Source: CAD feature listing. Evaluate the final solid. Frame: model axes, mm. A direction names the side the tool comes from. Round coordinates to 2 decimals unless told otherwise and drop trailing zeros. Loops run counter-clockwise (first coordinate to the right, second up) from the corner with the lowest first, then second, coordinate; pieces in that order, holes last. Notation, with made-up numbers: M 3,22.25 L 62,22.25 A13 cw 62,44.25 Z; hole C 34.5,16.25 d10. An arc over 180 degrees is marked long. Answer as CSV lines item,"result". Start each with the question number.
```python
from build123d import *

# Parameters (mm, degrees)
SKETCH1_W           = 10
SKETCH1_H           = 15.2
BOSS_EXTRUDE1_DEPTH = 1
SKETCH1_8_W         = 10
SKETCH1_8_H         = 15.2
SKETCH1_8_W_2       = 8.44
SKETCH1_8_H_2       = 13.64
BOSS_EXTRUDE2_DEPTH = 1
SKETCH1_9_RX        = 6.016925947
SKETCH1_9_RY        = 3.157568793
BOSS_EXTRUDE3_DEPTH = 0.5
FILLET1_R           = 2


with BuildPart() as part:
    # Sketch1 (on Front Plane) → Boss-Extrude1 (new body)
    with BuildSketch(Plane.XY):
        with Locations((5, 7.6)):
            Rectangle(SKETCH1_W, SKETCH1_H)
    extrude(amount=BOSS_EXTRUDE1_DEPTH)

    # Sketch1<8> (on Front Plane) → Boss-Extrude2 (add)
    with BuildSketch(Plane.XY):
        with Locations((5, 7.6)):
            Rectangle(SKETCH1_8_W, SKETCH1_8_H)
        with Locations((5, 7.6)):
            Rectangle(SKETCH1_8_W_2, SKETCH1_8_H_2, mode=Mode.SUBTRACT)
    extrude(amount=-BOSS_EXTRUDE2_DEPTH)

    # Sketch1<9> (on Front Plane) → Boss-Extrude3 (add)
    # profile 1 of 3: a face of its own
    with BuildSketch(Plane.XY):
        with Locations(Location((5, 7.6), (0, 0, -120.316314342))):
            Ellipse(SKETCH1_9_RX, SKETCH1_9_RY)
        with BuildLine():
            Line((5.55192436, 7.939742657), (5.714255538, 7.749614835))
            ThreePointArc((5.714255538, 7.749614835), (5.903370184, 7.16725844), (5.625306277, 6.621746036))
            Line((5.625306277, 6.621746036), (4.673505596, 5.809098397))
            Line((4.673505596, 5.809098397), (5.102260043, 5.306926538))
            Line((5.102260043, 5.306926538), (3.276812461, 5.306926538))
            Line((3.276812461, 5.306926538), (3.562960201, 7.109807107))
            Line((3.562960201, 7.109807107), (3.991714649, 6.607635249))
            Line((3.991714649, 6.607635249), (5.55192436, 7.939742657))
        make_face(mode=Mode.SUBTRACT)
        with BuildLine():
            Line((4.44807564, 7.260257343), (4.285744462, 7.450385165))
            ThreePointArc((4.285744462, 7.450385165), (4.096629816, 8.03274156), (4.374693723, 8.578253964))
            Line((4.374693723, 8.578253964), (5.326494404, 9.390901603))
            Line((5.326494404, 9.390901603), (4.897739957, 9.893073462))
            Line((4.897739957, 9.893073462), (6.723187539, 9.893073462))
            Line((6.723187539, 9.893073462), (6.437039799, 8.090192893))
            Line((6.437039799, 8.090192893), (6.008285351, 8.592364751))
            Line((6.008285351, 8.592364751), (4.44807564, 7.260257343))
        make_face(mode=Mode.SUBTRACT)
    # profile 2 of 3: a face of its own
    with BuildSketch(Plane.XY):
        with BuildLine():
            add(Edge.make_bspline(
                [(9.22, 11.980450807), (5, 22.611600433), (0.78, 6.751239794)],
                knots=[2.731060957, 2.731060957, 2.731060957, 5.172488647, 5.172488647, 5.172488647], degree=2, weights=[1, 0.342975287, 1]))
            Line((9.22, 11.980450807), (9.22, 14.42))
            Line((9.22, 14.42), (0.78, 14.42))
            Line((0.78, 14.42), (0.78, 6.751239794))
        make_face()
        with BuildLine():
            Line((1.807963278, 12.267050426), (2.573541086, 12.912762773))
            Line((2.573541086, 12.912762773), (2.629548837, 12.846358141))
            ThreePointArc((2.629548837, 12.846358141), (2.72234926, 12.554615255), (2.581675695, 12.282702073))
            Line((2.581675695, 12.282702073), (2.125075804, 11.897591397))
            Line((2.125075804, 11.897591397), (2.341285421, 11.641246159))
            Line((2.341285421, 11.641246159), (1.436292724, 11.641246159))
            Line((1.436292724, 11.641246159), (1.578739925, 12.538825176))
            Line((1.578739925, 12.538825176), (1.807963278, 12.267050426))
        make_face(mode=Mode.SUBTRACT)
        with BuildLine():
            Line((2.79925212, 13.230809928), (2.013248175, 12.570380578))
            Line((2.013248175, 12.570380578), (1.941775235, 12.655443444))
            ThreePointArc((1.941775235, 12.655443444), (1.849520441, 12.947359327), (1.99070215, 13.219009018))
            Line((1.99070215, 13.219009018), (2.47045985, 13.622119038))
            Line((2.47045985, 13.622119038), (2.272289715, 13.857969409))
            Line((2.272289715, 13.857969409), (3.166035288, 13.857969409))
            Line((3.166035288, 13.857969409), (3.036644718, 12.948279301))
            Line((3.036644718, 12.948279301), (2.79925212, 13.230809928))
        make_face(mode=Mode.SUBTRACT)
    # profile 3 of 3: a face of its own
    with BuildSketch(Plane.XY):
        with BuildLine():
            Line((0.78, 0.78), (9.22, 0.78))
            Line((9.22, 0.78), (9.22, 8.448760206))
            add(Edge.make_bspline(
                [(1.745579435, 2.034365319), (6.736770522, -0.884158057), (9.22, 8.448760206)],
                knots=[0, 0, 0, 2.030895994, 2.030895994, 2.030895994], degree=2, weights=[1, 0.527239314, 1]))
            add(Edge.make_bspline(
                [(0.78, 3.219549193), (1.100794809, 2.411393361), (1.745579435, 2.034365319)],
                knots=[5.872653611, 5.872653611, 5.872653611, 6.283185307, 6.283185307, 6.283185307], degree=2, weights=[1, 0.979006832, 1]))
            Line((0.78, 3.219549193), (0.78, 0.78))
        make_face()
        with BuildLine():
            Line((7.056197058, 2.135669885), (7.291696407, 1.863373763))
            Line((7.291696407, 1.863373763), (8.063431346, 2.521185925))
            Line((8.063431346, 2.521185925), (8.112322941, 2.464655019))
            ThreePointArc((8.112322941, 2.464655019), (8.208731591, 2.174084541), (8.071438446, 1.900448977))
            Line((8.071438446, 1.900448977), (7.601212367, 1.493766963))
            Line((7.601212367, 1.493766963), (7.828929297, 1.230469263))
            Line((7.828929297, 1.230469263), (6.912689643, 1.230469263))
            Line((6.912689643, 1.230469263), (7.056197058, 2.135669885))
        make_face(mode=Mode.SUBTRACT)
        with BuildLine():
            Line((8.277665846, 2.828924058), (7.517372897, 2.16210975))
            Line((7.517372897, 2.16210975), (7.461453822, 2.225867947))
            ThreePointArc((7.461453822, 2.225867947), (7.36303426, 2.515763479), (7.498428218, 2.790343716))
            Line((7.498428218, 2.790343716), (7.969285134, 3.203308389))
            Line((7.969285134, 3.203308389), (7.7510695, 3.452115))
            Line((7.7510695, 3.452115), (8.654696366, 3.452115))
            Line((8.654696366, 3.452115), (8.51075838, 2.563155))
            Line((8.51075838, 2.563155), (8.277665846, 2.828924058))
        make_face(mode=Mode.SUBTRACT)
    extrude(amount=-BOSS_EXTRUDE3_DEPTH)

    # Fillet1
    fillet1_edges = [part.edges().sort_by_distance(p)[0] for p in [
        (0.78, 0.78, -0.75),
        (0.78, 14.42, -0.75),
        (9.22, 14.42, -0.75),
        (9.22, 0.78, -0.75),
        (0, 15.2, 0),
        (0, 0, 0),
        (10, 0, 0),
        (10, 15.2, 0),
    ]]
    fillet(fillet1_edges, radius=FILLET1_R)


solid = part.part
```
1) Section B-B, the plane z = 0.25. Return loops of the section in (x, y).
2) Section C-C, the plane x = 0.5. Return loops of the section in (y, z), and give its area (3 significant figures).
3) Mould query, pull axis Y, two halves, no side actions, for faces 3 (the flat face through (2, 12, 0)), 4 (the cylindrical face through (0.57, 14.6, -0.01)), 5 (the flat face through (7.6, 1.7, 0)), 6 (the flat face through (0.5, 7.6, -1)). Classes: pulls with the +Y half, pulls with the -Y half, needs draft (parallel to the pull), parting line crosses it, or undercut.
4) Section A-A, the plane z = -0.65. Return loops of the section in (x, y), and give its area (3 significant figures).
5) Contact query for a flat-ended pin moving along its axis: pin 1 Ø1 at (x, y) = (7.5, 1.5) entering from -Z. Output: stop coordinate, or through.
6) Ray query, line 1 along Y through (x, z) = (3, -0.7); line 2 along X through (y, z) = (9, -0.8); line 3 along Y through (x, z) = (5.5, -0.45). Return the intervals inside material, ascending.
7) Access query for faces 1 (the flat face through (0, 8, 0)), 2 (the flat face through (0.78, 6.5, -0.6)). Directions: +Z, -Z, +X, -X, +Y, -Y. A direction counts if a zero-diameter tool reaches every point of the face in a straight line with its end or side. Return the directions, or none.
Findings below:
1,outline,"M 0,2 A2 ccw 2,0 L 8,0 A2 ccw 10,2 L 10,13.2 A2 ccw 8,15.2 L 2,15.2 A2 ccw 0,13.2 Z"
2,outline,"M 0.68,-1 L 14.52,-1 L 14.52,1 L 0.68,1 Z"
2,area,"27.7 mm²"
3,face 3,"undercut"
3,face 4,"pulls with the +Y half"
3,face 5,"undercut"
3,face 6,"needs draft"
4,outline,"M 0,2 A2 ccw 2,0 L 8,0 A2 ccw 10,2 L 10,13.2 A2 ccw 8,15.2 L 2,15.2 A2 ccw 0,13.2 Z; hole M 0.78,2.78 A2 ccw 2.78,0.78 L 7.22,0.78 A2 ccw 9.22,2.78 L 9.22,12.42 A2 ccw 7.22,14.42 L 2.78,14.42 A2 ccw 0.78,12.42 Z"
4,area,"36.9 mm²"
5,pin 1,"z = -0.5"
6,line 1,"0 to 0.78, 14.42 to 15.2"
6,line 2,"0 to 0.78, 9.22 to 10"
6,line 3,"0 to 2.79, 3.32 to 6.51, 7.9 to 8.16, 9.89 to 12.56, 13.03 to 15.2"
7,face 1,"+Z, -Z, -X, +Y, -Y"
7,face 2,"-Z"
